from build123d import *

# Parameters (mm, degrees)
EXTRUDE_1_DEPTH          = 30
SKETCH_2_R               = 5
EXTRUDE_2_DEPTH          = 10
SKETCH_3_W               = 140
SKETCH_3_H               = 160
CUT_EXTRUDE_1_DEPTH      = 10
CUT_EXTRUDE_2_DEPTH      = 158.241851935
CUT_EXTRUDE_2_DEPTH_BACK = 158.241851935
SKETCH_4_R               = 7.5


with BuildPart() as part:
    # 草图1 → 凸台-拉伸1 (new body)
    with BuildSketch(Plane.XY):
        with BuildLine():
            Line((-80, -95), (80, -95))
            ThreePointArc((80, -95), (87.071067812, -92.071067812), (90, -85))
            Line((90, -85), (90, 85))
            ThreePointArc((90, 85), (87.071067812, 92.071067812), (80, 95))
            Line((80, 95), (-80, 95))
            ThreePointArc((-80, 95), (-87.071067812, 92.071067812), (-90, 85))
            Line((-90, 85), (-90, -85))
            ThreePointArc((-90, -85), (-87.071067812, -92.071067812), (-80, -95))
        make_face()
    extrude(amount=EXTRUDE_1_DEPTH)

    # 草图2 → 凸台-拉伸2 (add)
    with BuildSketch(Plane(origin=(0, 0, 0), x_dir=(-1, 0, 0), z_dir=(0, 0, -1))):
        with BuildLine():
            Line((-95, -110), (95, -110))
            ThreePointArc((95, -110), (102.071067812, -107.071067812), (105, -100))
            Line((105, -100), (105, 100))
            ThreePointArc((105, 100), (102.071067812, 107.071067812), (95, 110))
            Line((95, 110), (-95, 110))
            ThreePointArc((-95, 110), (-102.071067812, 107.071067812), (-105, 100))
            Line((-105, 100), (-105, -100))
            ThreePointArc((-105, -100), (-102.071067812, -107.071067812), (-95, -110))
        make_face()
        with Locations((97.5, 0)):
            Circle(SKETCH_2_R, mode=Mode.SUBTRACT)
        with Locations((0, 102.5)):
            Circle(SKETCH_2_R, mode=Mode.SUBTRACT)
        with Locations((60, 102.5)):
            Circle(SKETCH_2_R, mode=Mode.SUBTRACT)
        with Locations((97.5, 50)):
            Circle(SKETCH_2_R, mode=Mode.SUBTRACT)
        with Locations(Location((97.5, -50, 0), (0, 0, 180))):
            Circle(SKETCH_2_R, mode=Mode.SUBTRACT)
        with Locations(Location((60, -102.5, 0), (0, 0, 180))):
            Circle(SKETCH_2_R, mode=Mode.SUBTRACT)
        with Locations(Location((0, -102.5, 0), (0, 0, 180))):
            Circle(SKETCH_2_R, mode=Mode.SUBTRACT)
        with Locations(Location((-60, 102.5, 0), (0, 0, 180))):
            Circle(SKETCH_2_R, mode=Mode.SUBTRACT)
        with Locations((-60, -102.5)):
            Circle(SKETCH_2_R, mode=Mode.SUBTRACT)
        with Locations((-97.5, -50)):
            Circle(SKETCH_2_R, mode=Mode.SUBTRACT)
        with Locations(Location((-97.5, 0, 0), (0, 0, 180))):
            Circle(SKETCH_2_R, mode=Mode.SUBTRACT)
        with Locations(Location((-97.5, 50, 0), (0, 0, 180))):
            Circle(SKETCH_2_R, mode=Mode.SUBTRACT)
    extrude(amount=EXTRUDE_2_DEPTH)

    # 草图3 → 切除-拉伸1 (cut)
    with BuildSketch(Plane(origin=(0, 0, -10), x_dir=(-1, 0, 0), z_dir=(0, 0, -1))):
        Rectangle(SKETCH_3_W, SKETCH_3_H)
    extrude(amount=-CUT_EXTRUDE_1_DEPTH, mode=Mode.SUBTRACT)

    # 草图4 → 切除-拉伸2 (cut, two sides: drawn at the far end of the back side and taken through both)
    with BuildSketch(Plane.XY.offset(30).offset(-CUT_EXTRUDE_2_DEPTH_BACK)):
        with Locations(Location((40, 45, 0), (0, 0, 180))):
            Circle(SKETCH_4_R)
        with Locations(Location((40, 0, 0), (0, 0, 180))):
            Circle(SKETCH_4_R)
        with Locations(Location((-45, 0, 0), (0, 0, 180))):
            Circle(SKETCH_4_R)
        with Locations(Location((-45, 65, 0), (0, 0, 180))):
            Circle(SKETCH_4_R)
        with Locations(Location((-45, -60, 0), (0, 0, 180))):
            Circle(SKETCH_4_R)
    extrude(amount=CUT_EXTRUDE_2_DEPTH + CUT_EXTRUDE_2_DEPTH_BACK, mode=Mode.SUBTRACT)


solid = part.part
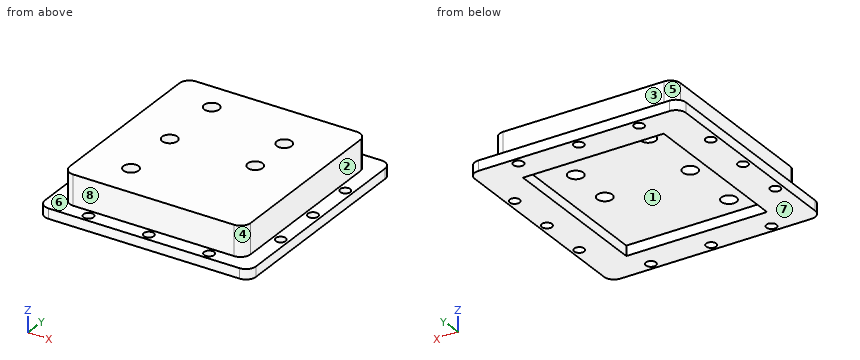
Can you work these out from the model? Positions are in its coordinate system, mm. Face numbers are marked on the shaded views. A direction names the side the tool comes from. Give positions to 0.01 mm unless a question says otherwise; leave off trailing zeros. Loops run counter-clockwise (first coordinate to the right, second up) from the corner with the lowest first, then second, coordinate; pieces in that order, holes last. Notation, with made-up numbers: (59, -28) -> (70, -28) arc R21 ccw to (70, 2) -> close; hole circle Ø9 at (45.5, -27). An arc over 180 degrees is marked (long way). Return JSON: item names as keys, results as strings.
Q1. We'd pull the mould along X, two halves only. Please class the marked faces 1, 2 and 3: released by +X, released by -X, zero draft, split by the parting line, or undercut.
Checks:
{"face 1": "undercut", "face 2": "released by +X", "face 3": "zero draft"}
Q2. I want a section at A-A, the plane x = -45. List the corners of the cut face in (y, z) for me, then the cut area to 3 significant figures.
Checks:
{"outline": "(-110, -10) -> (-80, -10) -> (-80, 0) -> (-67.5, 0) -> (-67.5, 30) -> (-95, 30) -> (-95, 0) -> (-110, 0) -> close; (-52.5, 0) -> (-7.5, 0) -> (-7.5, 30) -> (-52.5, 30) -> close; (7.5, 0) -> (57.5, 0) -> (57.5, 30) -> (7.5, 30) -> close; (72.5, 0) -> (80, 0) -> (80, -10) -> (110, -10) -> (110, 0) -> (95, 0) -> (95, 30) -> (72.5, 30) -> close", "area": "4,950 mm2"}
Q3. I want a section at D-D, the plane y = -15. List the corners of the cut face in (x, z) for me.
Checks:
{"outline": "(-105, -10) -> (-70, -10) -> (-70, 0) -> (70, 0) -> (70, -10) -> (105, -10) -> (105, 0) -> (90, 0) -> (90, 30) -> (-90, 30) -> (-90, 0) -> (-105, 0) -> close"}
Q4. For pin 1 Ø6 at (x, z) = (-75.5, 20) entering from -Y; pin 2 Ø9 at (x, y) = (-97.5, -50) entering from -Z; pin 3 Ø12 at (y, z) = (17, 23) entering from +X; pin 4 Ø4 at (y, z) = (69.5, 7) entering from -X, each with a flat end and sliding along its axis, tell me the tip position at first contact or that it passes through.
Checks:
{"pin 1": "stops at y = -95", "pin 2": "passes through", "pin 3": "stops at x = 90", "pin 4": "stops at x = -90"}
Q5. I want a section at C-C, the plane x = 60. List the corners of the cut face in (y, z) for me, then the cut area to 3 significant figures.
Checks:
{"outline": "(-110, -10) -> (-107.5, -10) -> (-107.5, 0) -> (-110, 0) -> close; (-97.5, -10) -> (-80, -10) -> (-80, 0) -> (80, 0) -> (80, -10) -> (97.5, -10) -> (97.5, 0) -> (95, 0) -> (95, 30) -> (-95, 30) -> (-95, 0) -> (-97.5, 0) -> close; (107.5, -10) -> (110, -10) -> (110, 0) -> (107.5, 0) -> close", "area": "6,100 mm2"}
Q6. On a 3-axis mill with a long thin cutter (end or side, diameter ignored), from which of +Z, -Z, +X, -X, +Y, -Y can I reach the whole of each face in a straight line? I mean the marked faces 4, 5, 6, 7 and 8. Say none if no direction works.
Checks:
{"face 4": "+Z, +X, -Y", "face 5": "+Z, -X, +Y", "face 6": "+Z", "face 7": "-Z, +X, -X, +Y, -Y", "face 8": "+Z, +X, -X, -Y"}
Q7. I want a section at B-B, the plane z = -6. Count the separate pieces of the cut face and the enclosed holes in it, then the cut area to 3 significant figures.
Checks:
{"separate pieces": "1", "enclosed holes": "13", "area": "22,800 mm2"}
Q8. I need wall thicknesses on probe 1 along Y at (x, z) = (-45, 12); probe 2 along Y at (x, z) = (60, -4.75); probe 3 along X at (y, z) = (65.5, -1). Which ranges of each line are inside material? Lowest first, please.
Checks:
{"probe 1": "y = -95 to -67.5, -52.5 to -7.5, 7.5 to 57.5, 72.5 to 95", "probe 2": "y = -110 to -107.5, -97.5 to -80, 80 to 97.5, 107.5 to 110", "probe 3": "x = -105 to -70, 70 to 105"}
